Input: part model. Units: mm. Frame: model coordinates. A direction names the side the tool comes from. Give positions to 0.01 mm unless a question says otherwise; leave off trailing zeros. Write each loop counter-clockwise with the first axis right and the second up, starting at its lowest first coordinate (ties: lowest second). Pieces come first, ordered by that corner, then holes. Notation, with made-up numbers: (63, 30) - (83, 30) arc R23 cw to (83, 57) - close; hole circle Ø11 at (-1.5, -6). An arc over 180 degrees is marked (long way). Answer as a JSON object with one key per item and string values. Group by question number.
from build123d import *

# Parameters (mm, degrees)
SKETCH1_W                   = 45
SKETCH1_H                   = 15
BOSS_EXTRUDE1_DEPTH         = 60
SHELL1_T                    = -4
SHELL1_THICKNESS_2_FACE_W   = 7
SHELL1_THICKNESS_2_FACE_H   = 37
SHELL1_THICKNESS_2_DEPTH    = 2
CUT_EXTRUDE3_REACH          = 67.812
SKETCH4_W                   = 10
SKETCH4_H                   = 10
SKETCH5_W                   = 7.4
SKETCH5_H                   = 7.4
CUT_EXTRUDE4_DEPTH          = 76.374067158
CUT_EXTRUDE5_START          = -1.2
CUT_EXTRUDE5_DEPTH          = 3.6
CUT_EXTRUDE6_REACH          = 124.321
SKETCH7_R                   = 2.1
BODY_MOVE_COPY1_START       = -7.5
BODY_MOVE_COPY1_OUTLINE_W   = 10
BODY_MOVE_COPY1_OUTLINE_H   = 10
BODY_MOVE_COPY1_DEPTH       = 4
BODY_MOVE_COPY1_START_2     = 3.7
BODY_MOVE_COPY1_2_OUTLINE_W = 10
BODY_MOVE_COPY1_2_OUTLINE_H = 10
BODY_MOVE_COPY1_2_DEPTH     = 3.8
BODY_MOVE_COPY1_START_3     = 3.5
BODY_MOVE_COPY1_3_OUTLINE_W = 10
BODY_MOVE_COPY1_3_OUTLINE_H = 2.8
BODY_MOVE_COPY1_3_DEPTH     = 0.2


# Read off the part's stored shape, not the designer's step: Body-Move/Copy1
with BuildPart() as part:
    # Sketch1 → Boss-Extrude1 (new, symmetric)
    with BuildSketch(Plane(origin=(0, 0, 0), x_dir=(1, 0, 0), z_dir=(0, 1, 0))):
        Rectangle(SKETCH1_W, SKETCH1_H)
    extrude(amount=BOSS_EXTRUDE1_DEPTH, both=True)

    # Shell1
    shell1_openings = [part.faces().sort_by_distance(p)[0] for p in [
        (0, 60, 0),
    ]]
    offset(amount=SHELL1_T, openings=shell1_openings, kind=Kind.INTERSECTION)

    # Shell1 thickness 2 face (on inner face of the shell) → Shell1 thickness 2 (add)
    with BuildSketch(Plane(origin=(0, -56, 0), x_dir=(0, 0, -1), z_dir=(0, -1, 0))):
        Rectangle(SHELL1_THICKNESS_2_FACE_W, SHELL1_THICKNESS_2_FACE_H)
    extrude(amount=-SHELL1_THICKNESS_2_DEPTH)

    # Sketch4 → Cut-Extrude3 (cut, up to next)
    with BuildSketch(Plane.XY.offset(7.5), mode=Mode.PRIVATE) as cut_extrude3_sk1:
        with Locations((0, 45)):
            Rectangle(SKETCH4_W, SKETCH4_H)
    cut_extrude3_tool1 = extrude(cut_extrude3_sk1.sketch, amount=-CUT_EXTRUDE3_REACH, mode=Mode.PRIVATE) & part.part
    add(cut_extrude3_tool1.solids().sort_by_distance((0, 45, 7.5))[0], mode=Mode.SUBTRACT)

    # Sketch5 → Cut-Extrude4 (cut, through all)
    with BuildSketch(Plane(origin=(22.5, 0, 0), x_dir=(0, 0, -1), z_dir=(1, 0, 0))):
        with Locations((0, 43.5)):
            Rectangle(SKETCH5_W, SKETCH5_H)
    extrude(amount=-CUT_EXTRUDE4_DEPTH, mode=Mode.SUBTRACT)

    # Sketch6 → Cut-Extrude5 (cut)
    with BuildSketch(Plane.XZ.offset(60).offset(CUT_EXTRUDE5_START)):
        Polygon((-15, 4.272391992), (-18.7, 2.136195996), (-18.7, -2.136195996), (-15, -4.272391992), (-11.3, -2.136195996), (-11.3, 2.136195996), align=None)
        Polygon((11.3, 2.136195996), (15, 4.272391992), (18.7, 2.136195996), (18.7, -2.136195996), (15, -4.272391992), (11.3, -2.136195996), align=None)
    extrude(amount=-CUT_EXTRUDE5_DEPTH, mode=Mode.SUBTRACT)

    # Sketch7 → Cut-Extrude6 (cut, up to next)
    with BuildSketch(Plane.XZ.offset(60), mode=Mode.PRIVATE) as cut_extrude6_sk1:
        with Locations(Location((-15, 0, 0), (0, 0, 270))):
            Circle(SKETCH7_R)
    cut_extrude6_tool1 = extrude(cut_extrude6_sk1.sketch, amount=-CUT_EXTRUDE6_REACH, mode=Mode.PRIVATE) & part.part
    # Sketch7 → Cut-Extrude6 (cut, up to next)
    with BuildSketch(Plane.XZ.offset(60), mode=Mode.PRIVATE) as cut_extrude6_sk2:
        with Locations(Location((15, 0, 0), (0, 0, 90))):
            Circle(SKETCH7_R)
    cut_extrude6_tool2 = extrude(cut_extrude6_sk2.sketch, amount=-CUT_EXTRUDE6_REACH, mode=Mode.PRIVATE) & part.part
    add(cut_extrude6_tool1.solids().sort_by_distance((-15, -60, 0))[0], mode=Mode.SUBTRACT)
    add(cut_extrude6_tool2.solids().sort_by_distance((15, -60, 0))[0], mode=Mode.SUBTRACT)

    # Body-Move/Copy1 outline → Body-Move/Copy1 (cut)
    with BuildSketch(Plane.XY.offset(BODY_MOVE_COPY1_START)):
        with Locations((0, 45)):
            Rectangle(BODY_MOVE_COPY1_OUTLINE_W, BODY_MOVE_COPY1_OUTLINE_H)
    extrude(amount=BODY_MOVE_COPY1_DEPTH, mode=Mode.SUBTRACT)

    # Body-Move_Copy1 2 outline → Body-Move_Copy1 2 (add)
    with BuildSketch(Plane.XY.offset(BODY_MOVE_COPY1_START_2)):
        with Locations((0, 45)):
            Rectangle(BODY_MOVE_COPY1_2_OUTLINE_W, BODY_MOVE_COPY1_2_OUTLINE_H)
    extrude(amount=BODY_MOVE_COPY1_2_DEPTH)

    # Body-Move_Copy1 3 outline → Body-Move_Copy1 3 (add)
    with BuildSketch(Plane.XY.offset(BODY_MOVE_COPY1_START_3)):
        with Locations((0, 48.6)):
            Rectangle(BODY_MOVE_COPY1_3_OUTLINE_W, BODY_MOVE_COPY1_3_OUTLINE_H)
    extrude(amount=BODY_MOVE_COPY1_3_DEPTH)


solid = part.part
1) Reachability of faces 1 (the face through (5.3, 43.4, -3.7)), 2 (the face through (12.918, -59.408, -0.273)), 3 (the face through (-13.18, -57.03, -3.22)), 4 (the face through (0, 40, -6)), 5 (the face through (-18.5, -6, 0)) from +Z, -Z, +X, -X, +Y, -Y: full face, straight path, thin tool, end or side. Return the list, or none.
2) Cut plane C-C on y = 19. Return the cut outline in (x, z), and give its area (3 significant figures).
3) Cut plane D-D on z = -5.75. Return the cut outline in (x, y).
4) Cut plane A-A on z = 0. Count the separate pieces of the cut face and the enclosed holes in it, and give its area (3 significant figures).
5) Cut plane B-B on x = 1.5. Return the cut outline in (y, z).
6) Line query: line 1 along X through (y, z) = (-59.05, 0); line 2 along X through (y, z) = (-11, -3); line 3 along Y through (x, z) = (-11.5, -0.5). Output: solid intervals per line, ascending. Write a range as from..to.
7) Pin query (flat end, axial travel): P1, Ø8, axis at x = 13.5, z = -1, coming from the -Y side; P2, Ø2, axis at x = -9, z = -1, coming from the +Y side; P3, Ø2.5, axis at x = 15, z = 0, coming from the -Y side. Return the tip coordinate at first contact, or that it passes through.
8) Mould query, pull axis Y, two halves, no side actions, for faces 6 (the face through (0, 60, -5)), 7 (the face through (16.82, -57.03, 3.22)), 8 (the face through (18.5, -6, 0)). Classes: +Y half, -Y half, draft (parallel to the pull), parting line (faces both ways), or undercut.
Filled in:
{
 "1": {"face 1": "+X, -X", "face 2": "-Y", "face 3": "none", "face 4": "-Z", "face 5": "+Y"},
 "2": {"outline": "(-22.5, -7.5) - (22.5, -7.5) - (22.5, 7.5) - (-22.5, 7.5) - close; hole (-18.5, -3.5) - (18.5, -3.5) - (18.5, 3.5) - (-18.5, 3.5) - close", "area": "416 mm²"},
 "3": {"outline": "(-22.5, -60) - (22.5, -60) - (22.5, 60) - (-22.5, 60) - close; hole (-5, 40) - (5, 40) - (5, 50) - (-5, 50) - close"},
 "4": {"separate pieces": "3", "enclosed holes": "0", "area": "1,060 mm²"},
 "5": {"outline": "(-60, -7.5) - (40, -7.5) - (40, -3.7) - (39.8, -3.7) - (39.8, -3.5) - (-54, -3.5) - (-54, 3.5) - (39.8, 3.5) - (39.8, 3.7) - (47.2, 3.7) - (47.2, 3.5) - (60, 3.5) - (60, 7.5) - (-60, 7.5) - close; (50, -7.5) - (60, -7.5) - (60, -3.5) - (50, -3.5) - close"},
 "6": {"line 1": "x = -22.5..-17.1, -12.9..12.9, 17.1..22.5", "line 2": "x = -22.5..-18.5, 18.5..22.5", "line 3": "y = -60..-58.8, -55.2..-54"},
 "7": {"P1": "stops at y = -60", "P2": "stops at y = -54", "P3": "stops at y = -55.2"},
 "8": {"face 6": "+Y half", "face 7": "undercut", "face 8": "draft"}
}
